from build123d import *

# Parameters (mm, degrees)
F0_W     = 29
F0_H     = 40.5
F1_DEPTH = 18
F2_W     = 25
F2_H     = 36.5
F3_DEPTH = 17
F5_R     = 2.25
F6_DEPTH = 5
F7_R     = 1
F8_R     = 1


with BuildPart() as f1:
    # F0 (on Front) → F1 (new body)
    with BuildSketch(Plane.XZ):
        with Locations((14.5, 20.25)):
            Rectangle(F0_W, F0_H)
    extrude(amount=F1_DEPTH)

    # F2 (on face) → F3 (cut)
    with BuildSketch(Plane.XZ.offset(18)):
        with Locations((14.5, 20.25)):
            Rectangle(F2_W, F2_H)
    extrude(amount=-F3_DEPTH, mode=Mode.SUBTRACT)

    # F5 (on face) → F6 (join)
    with BuildSketch(Plane.XZ.offset(1)):
        with Locations((23.25, 34.4)):
            Circle(F5_R)
    extrude(amount=F6_DEPTH)

    # F7
    f7_edges = [f1.edges().sort_by_distance(p)[0] for p in [
        (0, -9, 0),
        (29, -9, 0),
        (0, -9, 40.5),
        (29, -9, 40.5),
    ]]
    fillet(f7_edges, radius=F7_R)

    # F8
    f8_edges = [f1.edges().sort_by_distance(p)[0] for p in [
        (21, -6, 34.4),
    ]]
    fillet(f8_edges, radius=F8_R)


solid = f1.part
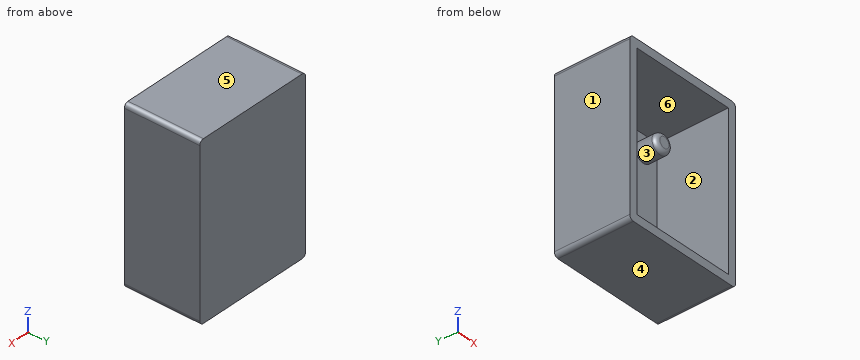
Source: CAD feature listing. Evaluate the final solid. Frame: model axes, mm. Face numbers are marked on the shaded views. A direction names the side the tool comes from. Give positions to 0.01 mm unless a question says otherwise; leave off trailing zeros. Write each loop counter-clockwise with the first axis right and the second up, starting at its lowest first coordinate (ties: lowest second). Pieces come first, ordered by that corner, then holes. Notation, with made-up numbers: M -26,58 L -6,58 A19 cw -6,90 Z; hole C 82.5,32.25 d8. An arc over 180 degrees is marked long. Return JSON: item names as keys, results as strings. Group by question number.
1) First-contact query: pin 1 Ø2 at (x, z) = (23, 11.5) entering from -Y; pin 2 Ø6 at (x, z) = (14.5, 8.5) entering from +Y; pin 3 Ø1.2 at (x, z) = (23.5, 34) entering from -Y. Flat tips, straight axial feed; report the tip coordinate or a pass-through.
2) Cut plane D-D, the plane z = 34.4. Output: boundary loops of the cut face in (x, y), then the cut area to 3 significant figures.
3) Ray query, L1, parallel to Z at x = 23.25, y = -2; L2, parallel to Z at x = 5.25, y = -7.75; L3, parallel to X at y = -6.25, z = 36.5. Return the intervals inside material, ascending.
4) Draft query along Z for the marked faces 3, 4, 5 and 6. Return one class per face: released by +Z, released by -Z, zero draft, split by the parting line, or undercut.
5) Cut plane C-C, the plane x = 23.25. Output: boundary loops of the cut face in (y, z), then the cut area to 3 significant figures.
6) Cut plane B-B, the plane z = 8.5. Output: boundary loops of the cut face in (x, y).
7) Set-up query: the marked faces 1 and 2. Return all of +Z, -Z, +X, -X, +Y, -Y with unobstructed straight access to the full face (end or side cutting, diameter ignored); none if empty.
8) Cut plane A-A, the plane y = -9.75. Output: boundary loops of the cut face in (x, z).
Data:
{
 "1": {"pin 1": "stops at y = -1", "pin 2": "stops at y = 0", "pin 3": "stops at y = -6"},
 "2": {"outline": "M 0,-18 L 2,-18 L 2,-1 L 21,-1 L 21,-5 A1 ccw 22,-6 L 24.5,-6 A1 ccw 25.5,-5 L 25.5,-1 L 27,-1 L 27,-18 L 29,-18 L 29,0 L 0,0 Z", "area": "119 mm²"},
 "3": {"L1": "z = 0 to 2, 32.15 to 36.65, 38.5 to 40.5", "L2": "z = 0 to 2, 38.5 to 40.5", "L3": "x = 0 to 2, 27 to 29"},
 "4": {"face 3": "undercut", "face 4": "released by -Z", "face 5": "released by +Z", "face 6": "undercut"},
 "5": {"outline": "M -18,0 L 0,0 L 0,40.5 L -18,40.5 L -18,38.5 L -1,38.5 L -1,36.65 L -5,36.65 A1 ccw -6,35.65 L -6,33.15 A1 ccw -5,32.15 L -1,32.15 L -1,2 L -18,2 Z", "area": "131 mm²"},
 "6": {"outline": "M 0,-18 L 2,-18 L 2,-1 L 27,-1 L 27,-18 L 29,-18 L 29,0 L 0,0 Z"},
 "7": {"face 1": "+Z, -Z, -X, +Y, -Y", "face 2": "-Y"},
 "8": {"outline": "M 0,1 A1 ccw 1,0 L 28,0 A1 ccw 29,1 L 29,39.5 A1 ccw 28,40.5 L 1,40.5 A1 ccw 0,39.5 Z; hole M 2,2 L 27,2 L 27,38.5 L 2,38.5 Z"}
}
